Design review of the part built by this model. Coordinates are the model's own, in mm. A direction names the side the tool comes from. Coordinates: 2 decimals unless noted, no trailing zeros. Write each loop counter-clockwise with the first axis right and the second up, starting at its lowest first coordinate (ties: lowest second). Pieces come first, ordered by that corner, then holes.
Q1. Add section B-B, the plane x = -65. Give the boundary of the cut face in (y, z).
Q2. Clearance check with flat-ended pins moving along their axes: pin 1 Ø10 at (x, y) = (9, 5.5) entering from +Z; pin 2 Ø3.5 at (y, z) = (38.5, -77.5) entering from +X; pin 3 Ø4.5 at (y, z) = (3.5, -106.5) entering from -X; pin 4 Ø7 at (x, z) = (0, 125) entering from -Y. State where each tip first meets the part, or that it passes through.
Q3. Add section C-C, the plane z = -137.5. Give the boundary of the cut face in (x, y), plus the area to 3 significant figures.
Q4. To check wall thickness, follow probe 1 along X at (y, z) = (103.65, 0) (3 decimals); probe 2 along Y at (x, z) = (88.5, -48.5); probe 3 along X at (y, z) = (98, 73). State the ranges of each line that lie inside material, in increasing order.
Q5. Machinability: for faces 1 (the face through (48.3, 5, -106)), 2 (the face through (39.645, 4.93, -113.262)), 3 (the face through (24.93, 57.082, 112.265)), which of the approach directions +Z, -Z, +X, -X, +Y, -Y give a long, thin tool a straight path to every point of the face, cutting with its end or side? Answer none if there is none.
Q6. Add section D-D, the plane y = 79.5. Give the boundary of the cut face in (x, z) (1 decimal), plus the area to 3 significant figures.
Q7. The part is to be moulded in two halves that separate along X. For faces 4 (the face through (91, 0, -67)), 5 (the face through (-39.887, 4.93, -113.177)), 6 (the face through (-32.5, 5, -144)), say which applies: +X half, -X half, draft (parallel to the pull), parting line (faces both ways), or undercut.
Q8. Add section A-A, the plane z = 0. Give the boundary of the cut face in (x, y) (1 decimal), plus the area to 3 significant figures.
Autodesk Inventor part; units mm, degrees
ref_plane "YZ Plane" through (0, 0, 0) normal (1, 0, 0) x (0, 1, 0)
ref_plane "XZ Plane" through (0, 0, 0) normal (0, 1, 0) x (-1, 0, 0)
ref_plane "XY Plane" through (0, 0, 0) normal (0, 0, 1) x (1, 0, 0)
sketch "Sketch1" plane through (0, 0, 0) normal (0, 1, 0) x (-1, 0, 0)
  circle A0 centre (0, 0) radius 135
  circle A1 centre (0, 0) radius 115
  circle A2 centre (0, 0) radius 112.0375
  circle A3 centre (0, 0) radius 9.5
  dimension "Absolute_Diameter" = 270
  dimension "Diameter_No_Outer_Lip" = 230
  dimension "Inner_Cylinder_Diameter" = 224.075
  dimension "Lip_Diameter" = 19
extrude "Extrusion1" add sketch "Sketch1" along normal blind 10 contours A0
extrude "Extrusion2" add sketch "Sketch1" along normal blind 105.5 contours A1
sketch "Sketch2" plane through (0, 105.5, 0) normal (0, 1, 0) x (1, 0, 0)
  circle A0 centre (0, 0) radius 115
  circle A1 centre (0, 0) radius 53.125
  dimension "Lip_Diameter_Out" = 230
  dimension "Inner_Lip_Diameter" = 106.25
extrude "Extrusion7" add sketch "Sketch2" against normal blind 5
sketch "Sketch24" plane through (0, 0, 0) normal (0, -1, 0) x (1, 0, 0)
  circle A0 centre (0, 0) radius 112.0375
  arc A1 (-85.157, -104.7535) -> (32.5, -131.0296) centre (0, 0) ccw
  circle A2 centre (0, 0) radius 133
  line L0 (-32.5, -70.125) -> (32.5, -70.125)
  line L1 (32.5, -70.125) -> (32.5, -160.125)
  line L2 (32.5, -160.125) -> (-32.5, -160.125)
  line L3 (-32.5, -160.125) -> (-32.5, -70.125)
  line L4 (-31, -158.625) -> (31, -158.625)
  line L5 (31, -158.625) -> (31, -71.625)
  line L6 (31, -71.625) -> (-31, -71.625)
  line L7 (-31, -71.625) -> (-31, -158.625)
  line L8 (-85.157, -65.125) -> (-46.3, -65.125)
  line L9 (-46.3, -65.125) -> (-46.3, -151.2985)
  line L10 (-46.3, -151.2985) -> (-85.157, -151.2985)
  line L11 (-85.157, -151.2985) -> (-85.157, -65.125)
  arc A3 (32.5, -131.0296) -> (-85.157, -104.7535) centre (0, 0) ccw
  line L12 (0, -71.625) -> (0, -158.625)
  line L13 (-83.157, -149.2985) -> (-48.3, -149.2985)
  line L14 (-48.3, -149.2985) -> (-48.3, -67.125)
  line L15 (-48.3, -67.125) -> (-83.157, -67.125)
  line L16 (-83.157, -67.125) -> (-83.157, -149.2985)
  line L17 (85.157, -65.125) -> (46.3, -65.125)
  line L18 (46.3, -65.125) -> (46.3, -151.2985)
  line L19 (46.3, -151.2985) -> (85.157, -151.2985)
  line L20 (85.157, -151.2985) -> (85.157, -65.125)
  line L21 (83.157, -149.2985) -> (48.3, -149.2985)
  line L22 (48.3, -149.2985) -> (48.3, -67.125)
  line L23 (48.3, -67.125) -> (83.157, -67.125)
  line L24 (83.157, -67.125) -> (83.157, -149.2985)
  circle A4 centre (0, 0) radius 120
  line L25 (-135, 0) -> (135, 0)
  point P0 (0, -135)
  point P1 (48.3, -126.0639)
  point P2 (83.157, -106.3481)
  point P3 (-31, -131.3925)
  point P4 (31, -131.3925)
  point P5 (-83.157, -106.3481)
  point P6 (-48.3, -126.0639)
  point P7 (46.3, -126.8121)
  point P8 (85.157, -104.7535)
  point P9 (-32.5, -131.0296)
  point P10 (-46.3, -126.8121)
  point P11 (48.3, -109.8504)
  point P12 (48.3, -101.0916)
  point P13 (31, -107.6634)
  point P14 (31, -115.9267)
  point P15 (-48.3, -109.8504)
  point P16 (-31, -115.9267)
  point P17 (-31, -107.6634)
  point P18 (-48.3, -101.0916)
  point P19 (83.157, -75.0821)
  point P20 (-83.157, -75.0821)
  point P21 (32.5, -115.5152)
  point P22 (-32.5, -115.5152)
  point P23 (31, -129.3368)
  point P24 (-31, -129.3368)
  dimension "d234" = 2
  dimension "d235" = 65
  dimension "d237" = 1.5
  dimension "d238" = 65.125
  dimension "d240" = 20.9625
  dimension "d241" = 270
  dimension "d242" = 70.125
  dimension "d243" = 13.8
  dimension "d244" = 38.857
  dimension "d247" = 2
  dimension "d248" = 90
  dimension "d253" = 240
extrude "Extrusion30" cut sketch "Sketch24" against normal up to surface (100.5 mm away) contours L24 A4 L22 A0 | A0 L22 L23 L24 | L16 L15 L14 A0 | A0 L14 A4 L16 | L24 A2 L22 A4 | A4 L14 A2 L16 | L24 A3 L22 A2 | A2 L14 A1 L16 | L5 A4 L12 A0 | A0 L12 L6 L5 | L7 L6 L12 A0 | A0 L12 A4 L7 | L5 A2 L12 A4 | A4 L12 A2 L7 | L5 A1 L12 A2 | A2 L12 A1 L7
extrude "Extrusion31" add sketch "Sketch24" against normal up to surface (10 mm away) contours L24 A4 L22 A0 | A0 L14 A4 L16 | L24 A2 L22 A4 | A4 L14 A2 L16 | L24 A3 L22 A2 | A2 L14 A1 L16 | L1 L2 L3 A1 L7 L4 L5
extrude "Extrusion32" cut sketch "Sketch24" against normal up to surface (100.5 mm away) contours L22 A4 L18 A0 | A0 L9 A4 L14 | L18 A4 L1 A0 | A0 L3 A4 L9 | L1 A4 L5 A0 | A0 L7 A4 L3
extrude "Extrusion35" add sketch "Sketch24" against normal blind 1 contours L1 A2 L5 A4 | A4 L7 A2 L3 | L1 A1 L5 A2 | A2 L7 A1 L3 | L5 A1 L12 A2 | L1 L2 L3 A1 L7 L4 L5 | A2 L12 A1 L7 | L5 L4 L12 A1 | A1 L12 L4 L7
fillet "Fillet19" radius 5 4 edges at (32.5, 0.5, -160.125) (31, 5.5, -158.625) (-32.5, 0.5, -160.125) (-31, 5.5, -158.625)
fillet "Fillet20" radius 2 4 edges at (-32.5, 5.5, -131.0296) (-32.5, 0.5, -131.0296) (32.5, 5.5, -131.0296) (32.5, 0.5, -131.0296)
sketch "Sketch27" plane through (0, 10, 0) normal (0, 1, 0) x (1, 0, 0)
  circle A0 centre (0, 0) radius 125
  circle A1 centre (0, 125) radius 2.75
  circle A2 centre (-73.4732, 101.1271) radius 2.75
  circle A3 centre (-118.8821, 38.6271) radius 2.75
  circle A4 centre (-118.8821, -38.6271) radius 2.75
  circle A5 centre (-73.4732, -101.1271) radius 2.75
  circle A6 centre (0, -125) radius 2.75
  circle A7 centre (73.4732, -101.1271) radius 2.75
  circle A8 centre (118.8821, -38.6271) radius 2.75
  circle A9 centre (118.8821, 38.6271) radius 2.75
  circle A10 centre (73.4732, 101.1271) radius 2.75
  dimension "d276" = 250
  dimension "d277" = 5.5
  dimension "d280" = 360
extrude "Extrusion36" cut sketch "Sketch27" against normal blind 10 contours A9 A0 | A0 A9 | A8 A0 | A0 A8 | A10 A0 | A0 A10 | A7 A0 | A0 A7 | A1 A0 | A0 A1 | A6 A0 | A0 A6 | A2 A0 | A0 A2 | A5 A0 | A0 A5 | A3 A0 | A0 A3 | A4 A0 | A0 A4
properties part number "Cylinder  Segment - 01"
Here are the results:
1. outline: (0, -118.32) - (10, -118.32) - (10, -91.25) - (0, -91.25) - close; (0, 91.25) - (100.5, 91.25) - (100.5, -94.87) - (105.5, -94.87) - (105.5, 94.87) - (10, 94.87) - (10, 118.32) - (0, 118.32) - close
2. pin 1: stops at z = 134.94
2. pin 2: stops at x = 86.53
2. pin 3: stops at x = -85.77
2. pin 4: stops at y = 0
3. outline: (-32.5, 0) - (32.5, 0) - (32.5, 10) - (31, 10) - (31, 1) - (-31, 1) - (-31, 10) - (-32.5, 10) - close
3. area: 92.0 mm2
4. probe 1: x = -115 to -53.125, 53.125 to 115
4. probe 2: y = 100.5 to 105.5
4. probe 3: x = -88.86 to -84.99, 84.99 to 88.86
5. face 1: -Y
5. face 2: +Y, -Y
5. face 3: +Y
6. outline: (-83.2, -79.4) - (-83.2, -75.1) arc R112 cw (long way) to (83.2, -75.1) - (83.2, -79.4) arc R115 ccw (long way) to start
6. area: 1,560 mm2
7. face 4: draft
7. face 5: undercut
7. face 6: -X half
8. outline: (-135, 0) - (-112, 0) - (-112, 100.5) - (-53.1, 100.5) - (-53.1, 105.5) - (-115, 105.5) - (-115, 10) - (-135, 10) - close; (53.1, 100.5) - (112, 100.5) - (112, 0) - (135, 0) - (135, 10) - (115, 10) - (115, 105.5) - (53.1, 105.5) - close
8. area: 1,610 mm2
